Autodesk Inventor part; units mm, degrees
ref_plane "YZ Plane" through (0, 0, 0) normal (1, 0, 0) x (0, 1, 0)
ref_plane "XZ Plane" through (0, 0, 0) normal (0, 1, 0) x (-1, 0, 0)
ref_plane "XY Plane" through (0, 0, 0) normal (0, 0, 1) x (1, 0, 0)
sketch "Sketch1" plane through (0, 0, 0) normal (0, 0, 1) x (1, 0, 0)
  line L0 (-152.4, -23.495) -> (152.4, -23.495)
  line L1 (152.4, -23.495) -> (152.4, 23.495)
  line L2 (152.4, 23.495) -> (-152.4, 23.495)
  line L3 (-152.4, 23.495) -> (-152.4, -23.495)
  line L4 (-152.4, -23.495) -> (152.4, 23.495) construction
  line L5 (152.4, -23.495) -> (-152.4, 23.495) construction
  point P0 (0, 0)
  dimension "d0" = 304.8
  dimension "d1" = 46.99
extrude "Extrusion1" add sketch "Sketch1" along normal blind 5.08
fillet "Fillet1" radius 12.7 4 edges at (152.4, 23.495, 2.54) (152.4, -23.495, 2.54) (-152.4, 23.495, 2.54) (-152.4, -23.495, 2.54)
sketch "Sketch2" plane through (0, 0, 5.08) normal (0, 0, 1) x (1, 0, 0)
  line L0 (-40.64, -20.32) -> (40.64, -20.32)
  line L1 (40.64, -20.32) -> (40.64, 20.32)
  line L2 (40.64, 20.32) -> (-40.64, 20.32)
  line L3 (-40.64, 20.32) -> (-40.64, -20.32)
  line L4 (-40.64, -20.32) -> (40.64, 20.32) construction
  line L5 (40.64, -20.32) -> (-40.64, 20.32) construction
  point P0 (0, 0)
  dimension "d5" = 81.28
  dimension "d6" = 40.64
sketch "Sketch3" plane through (0, 0, 5.08) normal (0, 0, 1) x (1, 0, 0)
  circle A0 centre (0, 12.7) radius 1.6891
  circle A1 centre (0, -12.7) radius 1.6891
  circle A2 centre (12.7, 0) radius 1.6891
  circle A3 centre (-12.7, 0) radius 1.6891
  circle A4 centre (0, 0) radius 4.699
  point P0 (0, 0)
  point P1 (0, 0)
  dimension "d7" = 3.3782
  dimension "d8" = 3.3782
  dimension "d9" = 3.3782
  dimension "d10" = 3.3782
  dimension "d11" = 9.398
  dimension "d12" = 12.7
  dimension "d13" = 12.7
  dimension "d14" = 12.7
  dimension "d15" = 12.7
  dimension "d16" = 0
extrude "Extrusion2" cut sketch "Sketch3" against normal blind 5.08
properties part number "New_Top"
Here's how the part is built. I have some questions about the finished solid (model axes, mm). Give positions to 0.01 mm unless a question says otherwise; leave off trailing zeros. Loops run counter-clockwise (first coordinate to the right, second up) from the corner with the lowest first, then second, coordinate; pieces in that order, holes last. Notation, with made-up numbers: M -18.5,22 L 40.5,22 A9 cw 40.5,38 Z; hole C -29.75,46 d10. An arc over 180 degrees is marked long. Return JSON: item names as keys, results as strings.
Item 1: Imagine slicing it at B-B on y = 19. List the corners of the cut face in (x, z) for me.
A:
{"outline": "M -149.39,0 L 149.39,0 L 149.39,5.08 L -149.39,5.08 Z"}
Item 2: Please list where these lines run through material, in increasing order: line 1 (Y direction, x = 0, z = 1.4) (3 decimals); line 2 (X direction, y = -3.5, z = 2.4); line 3 (X direction, y = -3, z = 0.6).
A:
{"line 1": "y = -23.495 to -14.389, -11.011 to -4.699, 4.699 to 11.011, 14.389 to 23.495", "line 2": "x = -152.4 to -3.14, 3.14 to 152.4", "line 3": "x = -152.4 to -3.62, 3.62 to 152.4"}
Item 3: Thinking about a two-plate mould opening in X: for faces 1 (the cylindrical face through (-0.61, 4.66, 2.58)), 2 (the cylindrical face through (-148.581, 19.873, 2.576)), 3 (the flat face through (152.4, 0, 3)), which applies, released by +X, released by -X, zero draft, split by the parting line, or undercut?
A:
{"face 1": "undercut", "face 2": "released by -X", "face 3": "released by +X"}
Item 4: Imagine slicing it at A-A on z = 3.8. List the corners of the cut face in (x, y) for me (3 decimals), then the cut area to 3 significant figures.
A:
{"outline": "M -152.4,-10.795 A12.7 ccw -139.7,-23.495 L 139.7,-23.495 A12.7 ccw 152.4,-10.795 L 152.4,10.795 A12.7 ccw 139.7,23.495 L -139.7,23.495 A12.7 ccw -152.4,10.795 Z; hole C -12.7,0 d3.378; hole C 0,0 d9.398; hole C 0,-12.7 d3.378; hole C 0,12.7 d3.378; hole C 12.7,0 d3.378", "area": "14,100 mm^2"}
Item 5: I'm going to push flat-ended pins straight in: pin 1 Ø2.5 at (x, y) = (-12.7, 0) entering from +Z; pin 2 Ø1 at (y, z) = (17, 2.5) entering from -X. Where does each tip first touch, or does it pass through?
A:
{"pin 1": "passes through", "pin 2": "stops at x = -151.05"}
